Work out the finished part from the listing and answer in its coordinate system (mm). Give positions to 0.01 mm unless a question says otherwise; leave off trailing zeros. Loops run counter-clockwise (first coordinate to the right, second up) from the corner with the lowest first, then second, coordinate; pieces in that order, holes last. Notation, with made-up numbers: (-16, 5) - (40, 5) arc R33 cw to (40, 35) - close; hole circle Ø9 at (52.25, 79). An arc over 180 degrees is marked (long way). One line per question, with ' | ' between items.
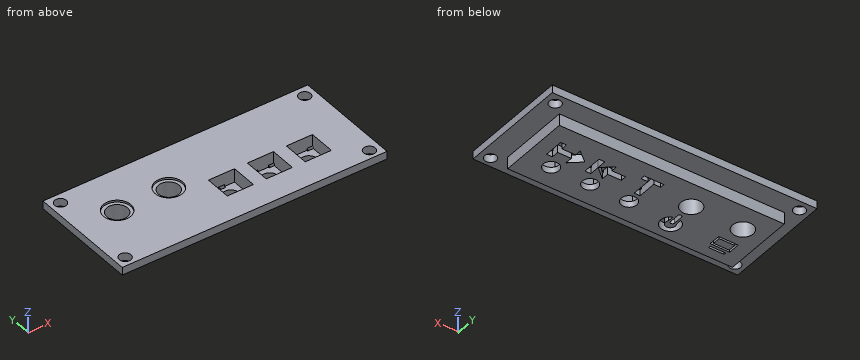
Autodesk Inventor part; units mm, degrees
ref_plane "YZ Plane" through (0, 0, 0) normal (1, 0, 0) x (0, 1, 0)
ref_plane "XZ Plane" through (0, 0, 0) normal (0, 1, 0) x (-1, 0, 0)
ref_plane "XY Plane" through (0, 0, 0) normal (0, 0, 1) x (1, 0, 0)
ref_plane "Work Plane1" through (0, 0, 0) normal (0, 0, 1) x (1, 0, 0)
sketch "Sketch1" plane through (0, 0, 0) normal (0, 0, 1) x (1, 0, 0)
  line L0 (67.7271, 45.3897) -> (135.6749, 45.3897)
  line L1 (135.6749, 45.3897) -> (135.6749, 17.2701)
  line L2 (135.6749, 17.2701) -> (67.7271, 17.2701)
  line L3 (67.7271, 17.2701) -> (67.7271, 45.3897)
  circle A0 centre (70.3236, 42.7621) radius 1.5
  circle A1 centre (70.2655, 19.7679) radius 1.5
  circle A2 centre (132.8977, 19.6632) radius 1.5
  circle A3 centre (132.9442, 42.6673) radius 1.5
  point P0 (0, 0)
  dimension "d0" = 3
  dimension "d1" = 3
  dimension "d2" = 3
  dimension "d3" = 3
extrude "Extrusion1" add sketch "Sketch1" along normal blind 2
sketch "Sketch2" plane through (0, 0, 0) normal (0, 0, -1) x (-1, 0, 0)
  line L0 (-130.1897, 21.9638) -> (-72.4709, 21.9638)
  line L1 (-72.4709, 21.9638) -> (-72.4709, 40.332)
  line L2 (-72.4709, 40.332) -> (-130.1897, 40.332)
  line L3 (-130.1897, 40.332) -> (-130.1897, 21.9638)
  point P0 (0, 0)
extrude "Extrusion2" add sketch "Sketch2" along normal blind 3
sketch "Sketch3" plane through (0, 0, -3) normal (0, 0, -1) x (-1, 0, 0)
  circle A0 centre (-123.1484, 27.6797) radius 2
  line L0 (-121.6186, 32.121) -> (-111.2555, 32.121)
  circle A1 centre (-113.1484, 27.6797) radius 2
  circle A2 centre (-103.1484, 27.6797) radius 2
  circle A3 centre (-91.5974, 33.7589) radius 2.65
  circle A4 centre (-78.3445, 33.7589) radius 2.65
  point P0 (0, 0)
  dimension "d8" = 4
  dimension "d11" = 10
  dimension "d16" = 5.3
  dimension "d17" = 5.3
extrude "Extrusion3" cut sketch "Sketch3" against normal up to surface (5 mm away)
sketch "Sketch5" plane through (0, 0, 2) normal (0, 0, 1) x (1, 0, 0)
  circle A0 centre (78.3445, 33.7589) radius 2.65
  circle A1 centre (78.3445, 33.7589) radius 3.5
  circle A2 centre (91.5974, 33.7589) radius 2.65
  circle A3 centre (91.5974, 33.7589) radius 3.5
  point P0 (0, 0)
  dimension "d22" = 7
  dimension "d23" = 7
extrude "Extrusion5" cut sketch "Sketch5" against normal blind 0.5
sketch "Sketch6" plane through (0, 0, 2) normal (0, 0, 1) x (1, 0, 0)
  line L0 (99.7984, 31.0297) -> (106.4984, 31.0297)
  line L1 (106.4984, 31.0297) -> (106.4984, 24.3297)
  line L2 (106.4984, 24.3297) -> (99.7984, 24.3297)
  line L3 (99.7984, 24.3297) -> (99.7984, 31.0297)
  circle A0 centre (103.1484, 27.6797) radius 2
  line L4 (109.7984, 31.0297) -> (116.4984, 31.0297)
  line L5 (116.4984, 31.0297) -> (116.4984, 24.3297)
  line L6 (116.4984, 24.3297) -> (109.7984, 24.3297)
  line L7 (109.7984, 24.3297) -> (109.7984, 31.0297)
  line L8 (119.7984, 31.0297) -> (126.4984, 31.0297)
  line L9 (126.4984, 31.0297) -> (126.4984, 24.3297)
  line L10 (126.4984, 24.3297) -> (119.7984, 24.3297)
  line L11 (119.7984, 24.3297) -> (119.7984, 31.0297)
  circle A1 centre (113.1484, 27.6797) radius 2
  circle A2 centre (123.1484, 27.6797) radius 2
  point P0 (0, 0)
  dimension "d26" = 6.7
  dimension "d27" = 6.7
  dimension "d28" = 3.35
  dimension "d29" = 3.35
  dimension "d30" = 6.7
  dimension "d31" = 6.7
  dimension "d32" = 6.7
  dimension "d33" = 6.7
  dimension "d34" = 3.35
  dimension "d35" = 3.35
  dimension "d36" = 3.35
  dimension "d37" = 3.35
extrude "Extrusion6" cut sketch "Sketch6" against normal blind 3.5
sketch "Sketch7" plane through (0, 0, -3) normal (0, 0, -1) x (-1, 0, 0)
  circle A0 centre (-103.1484, 27.6797) radius 2
  circle A1 centre (-91.5974, 33.7589) radius 2.65
  circle A2 centre (-123.1484, 27.6797) radius 2
  circle A3 centre (-78.3445, 33.7589) radius 2.65
  circle A4 centre (-113.1484, 27.6797) radius 2
  line L0 (-72.4709, 21.9638) -> (-130.1897, 21.9638)
  line L1 (-130.1897, 21.9638) -> (-130.1897, 40.332)
  line L2 (-130.1897, 40.332) -> (-72.4709, 40.332)
  line L3 (-72.4709, 40.332) -> (-72.4709, 21.9638)
  line L4 (-125.0325, 30.7395) -> (-126.5325, 30.7395)
  line L5 (-126.5325, 30.7395) -> (-126.5325, 35.7395)
  line L6 (-126.5325, 35.7395) -> (-125.0325, 35.7395)
  line L7 (-125.0325, 35.7395) -> (-125.0325, 34.1042)
  line L8 (-125.0325, 34.1042) -> (-121.5325, 34.1042)
  line L9 (-121.5325, 34.1042) -> (-121.5325, 35.7395)
  line L10 (-121.5325, 35.7395) -> (-118.5325, 33.2395)
  line L11 (-118.5325, 33.2395) -> (-121.5325, 30.7395)
  line L12 (-121.5325, 30.7395) -> (-121.5325, 32.6042)
  line L13 (-121.5325, 32.6042) -> (-125.0325, 32.6042)
  line L14 (-125.0325, 32.6042) -> (-125.0325, 30.7395)
  line L15 (-115.197, 30.7395) -> (-116.697, 30.7395)
  line L16 (-116.697, 30.7395) -> (-116.697, 35.7395)
  line L17 (-116.697, 35.7395) -> (-115.197, 35.7395)
  line L18 (-115.197, 35.7395) -> (-115.197, 33.3542)
  line L19 (-115.197, 33.3542) -> (-112.197, 35.7395)
  line L20 (-112.197, 35.7395) -> (-112.197, 34.1042)
  line L21 (-112.197, 34.1042) -> (-108.697, 34.1042)
  line L22 (-108.697, 34.1042) -> (-108.697, 32.6042)
  line L23 (-108.697, 32.6042) -> (-112.197, 32.6042)
  line L24 (-112.197, 32.6042) -> (-112.197, 30.7395)
  line L25 (-112.197, 30.7395) -> (-115.197, 33.3542)
  line L26 (-115.197, 33.3542) -> (-115.197, 30.7395)
  line L27 (-76.5, 25.1213) -> (-76.5, 24.561)
  line L28 (-76.5, 24.561) -> (-80.5, 24.561)
  line L29 (-80.5, 24.561) -> (-80.5, 25.1213)
  line L30 (-80.5, 25.1213) -> (-76.5, 25.1213)
  line L31 (-92.6211, 28.7032) -> (-92.6211, 27.1619)
  arc A5 (-92.6211, 27.1619) -> (-90.6211, 27.1619) centre (-91.6211, 26.4119) ccw
  line L32 (-90.6211, 27.1619) -> (-90.6211, 28.7032)
  arc A6 (-92.6211, 28.7032) -> (-90.6211, 28.7032) centre (-91.6211, 26.4119) ccw
  line L33 (-76.5, 26.3443) -> (-76.5, 28.3443)
  line L34 (-76.5, 28.3443) -> (-80.5, 28.3443)
  line L35 (-80.5, 28.3443) -> (-80.5, 26.3443)
  line L36 (-80.5, 26.3443) -> (-76.5, 26.3443)
  line L37 (-76, 28.8443) -> (-76, 25.8443)
  line L38 (-76, 25.8443) -> (-81, 25.8443)
  line L39 (-81, 25.8443) -> (-81, 28.8443)
  line L40 (-81, 28.8443) -> (-76, 28.8443)
  line L41 (-91.1211, 29.6705) -> (-91.1211, 27.1705)
  arc A7 (-92.1211, 27.1705) -> (-91.1211, 27.1705) centre (-91.6211, 27.1705) ccw
  line L42 (-92.1211, 27.1705) -> (-92.1211, 29.6705)
  arc A8 (-91.1211, 29.6705) -> (-92.1211, 29.6705) centre (-91.6211, 29.6705) ccw
  line L43 (-102.4368, 30.616) -> (-103.9441, 30.616)
  line L44 (-103.9441, 30.616) -> (-103.9441, 35.4734)
  line L45 (-103.9441, 35.4734) -> (-105.7188, 35.4734)
  line L46 (-105.7188, 35.4734) -> (-105.7188, 36.616)
  line L47 (-105.7188, 36.616) -> (-100.6621, 36.616)
  line L48 (-100.6621, 36.616) -> (-100.6621, 35.4734)
  line L49 (-100.6621, 35.4734) -> (-102.4368, 35.4734)
  line L50 (-102.4368, 35.4734) -> (-102.4368, 30.616)
  point P0 (0, 0)
extrude "Extrusion7" cut sketch "Sketch7" against normal blind 2 contours L4 L5 L6 L7 L8 L9 L10 L11 L12 L13 L14 | L19 L20 L21 L22 L23 L24 L25 | L15 L16 L17 L18 L26 | L27 L28 L29 L30 | L31 A5 L32 A6 | L37 L38 L39 L40 | L41 A7 L42 A8 | L43 L44 L45 L46 L47 L48 L49 L50
equation "\"d28\" = 0.5 * d26"
equation "\"d29\" = 0.5 * d27"
equation "\"d34\" = 0.5 * d31"
equation "\"d35\" = 0.5 * d33"
equation "\"d36\" = 0.5 * d30"
equation "\"d37\" = 0.5 * d32"
properties part number "InterfacePlate"
1. Find section D-D on y = 42. Write down the section's boundary in (x, z).
Evaluation:
outline: (67.73, 0) - (69.03, 0) - (69.03, 2) - (67.73, 2) - close; (71.62, 0) - (131.6, 0) - (131.6, 2) - (71.62, 2) - close; (134.29, 0) - (135.67, 0) - (135.67, 2) - (134.29, 2) - close
2. Find section C-C on z = 0.7. State how many separate pieces and enclosed holes the cut face has, then the cut area to 3 significant figures.
Evaluation:
separate pieces: 1 | enclosed holes: 9 | area: 1,700 mm2
3. Consider L1, parallel to X at y = 27.75, z = -0.55; L2, parallel to Y at x = 111, z = -0.05; L3, parallel to X at y = 34.75, z = -0.55. Determine where each line is inside the solid, lowest interval first.
Evaluation:
L1: 72.47 to 99.8, 106.5 to 109.8, 116.5 to 119.8, 126.5 to 130.19 | L2: 21.96 to 24.33, 31.03 to 40.33 | L3: 72.47 to 75.89, 80.8 to 89.14, 94.06 to 130.19
4. Flat-ended cylindrical pins translate along their axes: pin 1 (1.3 mm diameter, centred on y = 34.5, z = -2, fed in from -X); pin 2 (3 mm diameter, centred on y = 27, z = -2, fed in from +X); pin 3 (1 mm diameter, centred on x = 79, z = -1.5, fed in from -Y); pin 4 (5.5 mm diameter, centred on x = 114, y = 27.5, fed in from +Z). Find the tip coordinate at first contact, or state that the pin passes through.
Evaluation:
pin 1: x = 72.47 | pin 2: x = 130.19 | pin 3: y = 21.96 | pin 4: z = 2
5. Find section B-B on x = 128. Write down the section's boundary in (y, z).
Evaluation:
outline: (17.27, 0) - (21.96, 0) - (21.96, -3) - (40.33, -3) - (40.33, 0) - (45.39, 0) - (45.39, 2) - (17.27, 2) - close
6. Find section A-A on y = 38. Write down the section's boundary in (x, z), then the cut area to 3 significant figures.
Evaluation:
outline: (67.73, 0) - (72.47, 0) - (72.47, -3) - (130.19, -3) - (130.19, 0) - (135.67, 0) - (135.67, 2) - (67.73, 2) - close | area: 309 mm2
